Verification items for the finished model (mm, model axes). Face numbers are marked on the shaded views. A direction names the side the tool comes from. Round coordinates to 2 decimals unless told otherwise and drop trailing zeros. Write each loop counter-clockwise with the first axis right and the second up, starting at its lowest first coordinate (ties: lowest second). Pieces come first, ordered by that corner, then holes. Notation, with made-up numbers: (48, -18.5) - (79, -18.5) arc R30 cw to (79, 11.5) - close; hole circle Ø11 at (-26, 59). An arc over 180 degrees is marked (long way). Write each question's results on one line, items separated by ' | '.
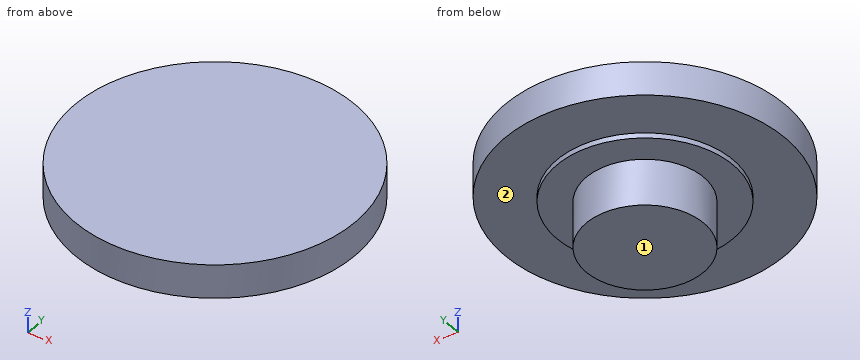
```python
from build123d import *

# Parameters (mm, degrees)
F0_R     = 9.55
F0_R_2   = 6
F1_DEPTH = 2.3
F0_R_3   = 4
F2_DEPTH = 2.65
F3_DEPTH = 5.8


with BuildPart() as f1:
    # F0 (on Top) → F1 (new body)
    with BuildSketch(Plane.XY):
        Circle(F0_R)
        Circle(F0_R_2, mode=Mode.SUBTRACT)
    extrude(amount=-F1_DEPTH)

    # F0 (on Top) → F2 (join)
    with BuildSketch(Plane.XY):
        Circle(F0_R_2)
        Circle(F0_R_3, mode=Mode.SUBTRACT)
    extrude(amount=-F2_DEPTH)

    # F0 (on Top) → F3 (join)
    with BuildSketch(Plane.XY):
        Circle(F0_R_3)
    extrude(amount=-F3_DEPTH)


solid = f1.part
```
(1) Section check A-A (x = 0). Record the cut outline in (y, z), plus the area to 3 significant figures.
Answer:
outline: (-9.55, -2.3) - (-6, -2.3) - (-6, -2.65) - (-4, -2.65) - (-4, -5.8) - (4, -5.8) - (4, -2.65) - (6, -2.65) - (6, -2.3) - (9.55, -2.3) - (9.55, 0) - (-9.55, 0) - close | area: 73.3 mm2
(2) Section check C-C (z = -2.9). Record the cut outline in (x, y), plus the area to 3 significant figures.
Answer:
outline: circle Ø8 at (0, 0) | area: 50.3 mm2
(3) Go/stop test with flat-tipped pins: pin 1 Ø1 at (y, z) = (-5.5, -3.5) entering from -X; pin 2 Ø1.5 at (x, z) = (5, -1.5) entering from +Y; pin 3 Ø1.5 at (x, z) = (-2, -3) entering from -Y. Record where each tip stops, or that it passes through.
Answer:
pin 1: through | pin 2: y = 8.55 | pin 3: y = -9.39
(4) Section check D-D (x = -4.5). Record the cut outline in (y, z), plus the area to 3 significant figures.
Answer:
outline: (-8.42, -2.3) - (-3.97, -2.3) - (-3.97, -2.65) - (3.97, -2.65) - (3.97, -2.3) - (8.42, -2.3) - (8.42, 0) - (-8.42, 0) - close | area: 41.5 mm2
(5) Thickness scan on L1, parallel to Z at x = -1, y = -5; L2, parallel to Z at x = 3.25, y = 6.75; L3, parallel to X at y = 0.5, z = -4.6. Record the ranges inside material, lowest first.
Answer:
L1: -2.65 to 0 | L2: -2.3 to 0 | L3: -3.97 to 3.97
(6) Set-up check for the marked faces 1 and 2: record each of +Z, -Z, +X, -X, +Y, -Y from which the full face is reachable in a straight line by a thin tool's end or side.
Answer:
face 1: -Z, +X, -X, +Y, -Y | face 2: -Z
